CAD build for the part. Positions are in the model's coordinates, mm. A direction names the side the tool comes from. Give positions to 0.01 mm unless a question says otherwise; leave off trailing zeros. Loops run counter-clockwise (first coordinate to the right, second up) from the corner with the lowest first, then second, coordinate; pieces in that order, holes last.
```python
from build123d import *

# Parameters (mm, degrees)
BOSS_EXTRUDE1_DEPTH = 6
BOSS_EXTRUDE2_DEPTH = 26.3
BOSS_EXTRUDE3_DEPTH = 6
SKETCH8_R           = 1.7
BOSS_EXTRUDE4_DEPTH = 3


with BuildPart() as part:
    # Sketch1 → Boss-Extrude1 (new body)
    with BuildSketch(Plane.XY):
        with BuildLine():
            Line((0, 0), (20, 0))
            Line((20, 0), (20, 4))
            Line((20, 4), (23.6, 4))
            Line((23.6, 4), (23.6, 11))
            Line((23.6, 11), (17.3, 11))
            ThreePointArc((17.3, 11), (9.3, 19), (1.3, 11))
            Line((1.3, 11), (-2.7, 11))
            Line((-2.7, 11), (-2.7, 4))
            Line((-2.7, 4), (0, 4))
            Line((0, 4), (0, 0))
        make_face()
        Polygon((11.118653348, 14.15), (7.481346652, 14.15), (5.662693304, 11), (7.481346652, 7.85), (11.118653348, 7.85), (12.937306696, 11), align=None, mode=Mode.SUBTRACT)
    extrude(amount=BOSS_EXTRUDE1_DEPTH)

    # Sketch2 → Boss-Extrude2 (add)
    with BuildSketch(Plane.ZY.offset(2.7)):
        with BuildLine():
            Line((6, 4), (6, 5))
            ThreePointArc((6, 5), (6.292893219, 4.292893219), (7, 4))
            Line((7, 4), (6, 4))
        make_face()
    extrude(amount=-BOSS_EXTRUDE2_DEPTH)

    # Sketch4 → Boss-Extrude3 (add)
    with BuildSketch(Plane.XY.offset(6)):
        with BuildLine():
            Line((23.1, 4), (23.1, 5))
            ThreePointArc((23.1, 5), (23.392893219, 4.292893219), (24.1, 4))
            Line((24.1, 4), (23.1, 4))
        make_face()
        with BuildLine():
            Line((-1.5, 4), (-2.5, 4))
            ThreePointArc((-2.5, 4), (-1.792893219, 4.292893219), (-1.5, 5))
            Line((-1.5, 5), (-1.5, 4))
        make_face()
    extrude(amount=-BOSS_EXTRUDE3_DEPTH)

    # Sketch8 → Boss-Extrude4 (add)
    with BuildSketch(Plane.XY.offset(6)):
        Polygon((7.452479139, 14.2), (5.604958277, 11), (7.452479139, 7.8), (11.147520861, 7.8), (12.995041723, 11), (11.147520861, 14.2), align=None)
        with Locations((9.3, 11)):
            Circle(SKETCH8_R, mode=Mode.SUBTRACT)
    extrude(amount=-BOSS_EXTRUDE4_DEPTH)


solid = part.part
```
1. Drop flat-ended pins along their axis: pin 1 (7 mm diameter, centred on x = 6, y = 15, fed in from +Z); pin 2 (3 mm diameter, centred on x = 19, z = 4, fed in from +Y); pin 3 (1.2 mm diameter, centred on y = 1.5, z = 4, fed in from +X). Give the stop position or say it passes through.
Responses:
pin 1: stops at z = 6
pin 2: stops at y = 11
pin 3: stops at x = 20
2. Tool access for faces 4 (the face through (6.559, 9.447, 1.479)), 5 (the face through (20, 11, 3)), 6 (the face through (-1, 11, 3)): list every direction of +Z, -Z, +X, -X, +Y, -Y with a clear straight run to the whole face (end or side of a thin tool).
Responses:
face 4: -Z
face 5: +Z, -Z, +X, +Y
face 6: +Z, -Z, -X, +Y
3. Pull direction X, two halves, no side cores. Call faces 1 (the face through (0, 2, 3)), 2 (the face through (10.214, 12.433, 4.521)), 3 (the face through (10.5, 7.5, 0)): released by +X, released by -X, zero draft, split by the parting line, or undercut.
Responses:
face 1: released by -X
face 2: undercut
face 3: zero draft
4. Saw through at D-D, the plane y = 11.5. List the corners of the cut face in (x, z).
Responses:
outline: (1.32, 0) - (5.95, 0) - (5.95, 3) - (7.68, 3) - (7.68, 6) - (1.32, 6) - close; (10.92, 3) - (12.65, 3) - (12.65, 0) - (17.28, 0) - (17.28, 6) - (10.92, 6) - close
5. Probe line 1 along Y through (x, z) = (9.3, 3.95); line 2 along Y through (x, z) = (20.5, 1.75); line 3 along Z through (x, y) = (19, 7.75). List the from-to ranges inside material, lowest first.
Responses:
line 1: y = 0 to 9.3, 12.7 to 19
line 2: y = 4 to 11
line 3: z = 0 to 6
6. Saw through at C-C, the plane x = 18. List the corners of the cut face in (y, z), and give its area (3 significant figures).
Responses:
outline: (0, 0) - (11, 0) - (11, 6) - (5, 6) arc R1 cw to (4, 7) - (4, 6) - (0, 6) - close
area: 66.2 mm2
7. Saw through at A-A, the plane x = 9.3. List the corners of the cut face in (y, z), and give its area (3 significant figures).
Responses:
outline: (0, 0) - (7.85, 0) - (7.85, 3) - (9.3, 3) - (9.3, 6) - (5, 6) arc R1 cw to (4, 7) - (4, 6) - (0, 6) - close; (12.7, 3) - (14.15, 3) - (14.15, 0) - (19, 0) - (19, 6) - (12.7, 6) - close
area: 85.1 mm2
8. Saw through at B-B, the plane z = 2. List the corners of the cut face in (x, y), and give its area (3 significant figures).
Responses:
outline: (-2.7, 4) - (0, 4) - (0, 0) - (20, 0) - (20, 4) - (24.1, 4) arc R1 cw to (23.6, 4.13) - (23.6, 11) - (17.3, 11) arc R8 ccw to (1.3, 11) - (-2.7, 11) - close; hole (5.66, 11) - (7.48, 7.85) - (11.12, 7.85) - (12.94, 11) - (11.12, 14.15) - (7.48, 14.15) - close
area: 330 mm2
